Geometry: final body of the model. Coordinates: model frame, mm. A direction names the side the tool comes from. Coordinates: 2 decimals unless noted, no trailing zeros. Loops run counter-clockwise (first coordinate to the right, second up) from the corner with the lowest first, then second, coordinate; pieces in that order, holes last. Notation, with made-up numbers: (-22, 21.5) - (-6, 21.5) arc R25 ccw to (-6, 55.5) - close; hole circle Ø9 at (6.5, 4.25). An arc over 180 degrees is marked (long way). Answer in a Markdown table with one row per item.
from build123d import *

# Parameters (mm, degrees)
SKETCH_W     = 46.736
SKETCH_H     = 34.544
PAD_DEPTH    = 4.064
SKETCH001_W  = 55.88
SKETCH001_H  = 34.544
PAD001_DEPTH = 1.778
SKETCH002_R  = 1.27
POCKET_DEPTH = 1.779
FILLET_R     = 1.524


with BuildPart() as part:
    # Sketch → Pad (new body)
    with BuildSketch(Plane.XZ):
        Rectangle(SKETCH_W, SKETCH_H)
    extrude(amount=PAD_DEPTH)

    # Sketch001 (on Face5 of Pad) → Pad001 (join)
    with BuildSketch(Plane(origin=(0, 0, 0), x_dir=(1, 0, 0), z_dir=(0, 1, 0))):
        Rectangle(SKETCH001_W, SKETCH001_H)
    extrude(amount=PAD001_DEPTH)

    # Sketch002 (on Face7 of Pad001) → Pocket (cut, through all)
    with BuildSketch(Plane.XZ):
        with Locations((25, 14.5)):
            Circle(SKETCH002_R)
        with Locations((-25, 14.5)):
            Circle(SKETCH002_R)
        with Locations((-25, -14.5)):
            Circle(SKETCH002_R)
        with Locations((25, -14.5)):
            Circle(SKETCH002_R)
    extrude(amount=-POCKET_DEPTH, mode=Mode.SUBTRACT)

    # Fillet
    fillet_edges = [part.edges().sort_by_distance(p)[0] for p in [
        (27.94, 0.889, -17.272),
        (27.94, 0.889, 17.272),
        (-27.94, 0.889, 17.272),
        (-27.94, 0.889, -17.272),
    ]]
    fillet(fillet_edges, radius=FILLET_R)


with BuildPart() as part_1:
    # Body placement: moved
    add(part.part.moved(Location((-3.273552, 2.72796, 0))))


solid = part_1.part
(1) Cut plane C-C on y = 1.15. Output: boundary loops of the cut face in (x, z).
Verdict:
| item | result |
|---|---|
| outline | (-26.64, -17.27) - (20.09, -17.27) - (20.09, 17.27) - (-26.64, 17.27) - close |
(2) Access query for faces 5 (the face through (22, 2.728, 0)), 6 (the face through (-31.214, 4, 0)), 7 (the face through (-26.642, 1, 0)). Directions: +Z, -Z, +X, -X, +Y, -Y. A direction counts if a zero-diameter tool reaches every point of the face in a straight line with its end or side. Return the directions, or none.
Verdict:
| item | result |
|---|---|
| face 5 | +Z, -Z, +X, -Y |
| face 6 | +Z, -Z, -X, +Y, -Y |
| face 7 | +Z, -Z, -X, -Y |
(3) Ray query, probe 1 along X at (y, z) = (1.15, 9.5). Return the intervals inside material, ascending.
Verdict:
| item | result |
|---|---|
| probe 1 | x = -26.64 to 20.09 |
(4) Cut plane B-B on z = 0.5. Output: boundary loops of the cut face in (x, y).
Verdict:
| item | result |
|---|---|
| outline | (-31.21, 2.73) - (-26.64, 2.73) - (-26.64, -1.34) - (20.09, -1.34) - (20.09, 2.73) - (24.67, 2.73) - (24.67, 4.51) - (-31.21, 4.51) - close |
(5) First-contact query: pin 1 Ø3 at (y, z) = (0.5, -3) entering from -X; pin 2 Ø1.5 at (x, z) = (21.73, -14.5) entering from -Y; pin 3 Ø1.4 at (x, z) = (21.5, -4) entering from -Y. Flat tips, straight axial feed; report the tip coordinate or a pass-through.
Verdict:
| item | result |
|---|---|
| pin 1 | stops at x = -26.64 |
| pin 2 | passes through |
| pin 3 | stops at y = 2.73 |
(6) Pull-direction query (X, two-part tool) for faces 1 (the face through (-4, 2, -17.272)), 2 (the face through (21.56, 3.6, -13.24)), 3 (the face through (-30.78, 3.63, 16.81)), 4 (the face through (21.56, 3.6, 15.76)); classes: pulls with the +X half, pulls with the -X half, needs draft (parallel to the pull), parting line crosses it, or undercut.
Verdict:
| item | result |
|---|---|
| face 1 | needs draft |
| face 2 | undercut |
| face 3 | pulls with the -X half |
| face 4 | undercut |
(7) Cut plane A-A on z = 14.5. Output: boundary loops of the cut face in (x, y).
Verdict:
| item | result |
|---|---|
| outline | (-31.21, 2.73) - (-29.54, 2.73) - (-29.54, 4.51) - (-31.21, 4.51) - close; (-27, 2.73) - (-26.64, 2.73) - (-26.64, -1.34) - (20.09, -1.34) - (20.09, 2.73) - (20.46, 2.73) - (20.46, 4.51) - (-27, 4.51) - close; (23, 2.73) - (24.67, 2.73) - (24.67, 4.51) - (23, 4.51) - close |
